```python
from build123d import *

# Parameters (mm, degrees)
SKETCH1_W           = 73.5
SKETCH1_H           = 5
BOSS_EXTRUDE1_DEPTH = 17
CUT_EXTRUDE1_DEPTH  = 195.359872402


with BuildPart() as part:
    # Sweep3: sweep along a path in Sketch2
    with BuildLine(Plane(origin=(0, 0, 0), x_dir=(0, 0, -1), z_dir=(1, 0, 0))) as sweep3_path:
        Line((-73.8, 0), (-73.8, 86.85))
        Line((-73.8, 86.85), (-63.15, 97.5))
        Line((-63.15, 97.5), (63.15, 97.5))
        Line((63.15, 97.5), (73.8, 86.85))
        Line((73.8, 86.85), (73.8, 0))
    # Sketch1 → Sweep3 (sweep)
    with BuildSketch(Plane(origin=(0, 0, 0), x_dir=(1, 0, 0), z_dir=(0, 1, 0))):
        with Locations((-13.25, -73.8)):
            Rectangle(SKETCH1_W, SKETCH1_H)
    sweep(path=sweep3_path.line, transition=Transition.RIGHT)

    # Sketch5 → Boss-Extrude1 (add)
    with BuildSketch(Plane.ZY.offset(50)):
        Polygon((-76.3, 0), (-71.3, 0), (-71.3, 85.814466094), (-62.114466094, 95), (62.114466094, 95), (71.3, 85.814466094), (71.3, 0), (76.3, 0), (76.3, 87.885533906), (64.185533906, 100), (-64.185533906, 100), (-76.3, 87.885533906), align=None)
    extrude(amount=BOSS_EXTRUDE1_DEPTH)

    # Sketch6 → Cut-Extrude1 (cut, through all)
    with BuildSketch(Plane(origin=(0, 0, -76.3), x_dir=(-1, 0, 0), z_dir=(0, 0, -1))):
        Polygon((52.03, 0), (67, 27), (67, 0), align=None)
    extrude(amount=-CUT_EXTRUDE1_DEPTH, mode=Mode.SUBTRACT)


solid = part.part
```
Geometry: final body of the model. Coordinates: model frame, mm. A direction names the side the tool comes from. Round coordinates to 2 decimals unless told otherwise and drop trailing zeros. Order: outer loops, then holes, each group sorted by start corner. A loop starts at its lowest first (then second) coordinate and runs counter-clockwise, first axis right, second up. Notation, with made-up numbers: M 35,-2.5 L 72,-2.5 A15 ccw 72,25.5 Z; hole C 10.25,-1 d8. An arc over 180 degrees is marked long. Use one line per item in the form item = value. Start each with the question number.
Q1. Access query for faces 1 (the face through (-21, 44, 71.3)), 2 (the face through (-21, 100, 1)). Directions: +Z, -Z, +X, -X, +Y, -Y. A direction counts if a zero-diameter tool reaches every point of the face in a straight line with its end or side. Return the directions, or none.
Q2. Material intervals for line 1 (Z direction, x = 4, y = 11); line 2 (Y direction, x = -10, z = 12); line 3 (Z direction, x = -34, y = 93), sorted ascending. Write a range as [from, to].
Q3. Cut plane C-C (y = 74). Return loops of the section in (x, z), and give its area (3 significant figures).
Q4. Cut plane D-D (z = 5). Return loops of the section in (x, y).
Q5. Cut plane B-B (x = -5). Return loops of the section in (y, z), and give its area (3 significant figures).
Q6. Cut plane A-A (y = 91.5). Return loops of the section in (x, z).
Q7. Mould query, pull axis Z, two halves, no side actions, for faces 3 (the face through (-21.117, 90.472, 66.643)), 4 (the face through (-21, 43, 76.3)), 5 (the face through (-59.41, 13.31, -73.83)). Classes: +Z half, -Z half, draft (parallel to the pull), parting line (faces both ways), or undercut.
Geometry results:
q1.face_1 = +X, -X, -Y
q1.face_2 = +Z, -Z, +X, -X, +Y
q2.line_1 = [-76.3, -71.3], [71.3, 76.3]
q2.line_2 = [95, 100]
q2.line_3 = [-71.19, -64.11], [64.11, 71.19]
q3.outline = M -67,-76.3 L 23.5,-76.3 L 23.5,-71.3 L -67,-71.3 Z; M -67,71.3 L 23.5,71.3 L 23.5,76.3 L -67,76.3 Z
q3.area = 905 mm^2
q4.outline = M -67,95 L 23.5,95 L 23.5,100 L -67,100 Z
q5.outline = M 0,-76.3 L 87.89,-76.3 L 100,-64.19 L 100,64.19 L 87.89,76.3 L 0,76.3 L 0,71.3 L 85.81,71.3 L 95,62.11 L 95,-62.11 L 85.81,-71.3 L 0,-71.3 Z
q5.area = 1,650 mm^2
q6.outline = M -67,-72.69 L 23.5,-72.69 L 23.5,-65.61 L -67,-65.61 Z; M -67,65.61 L 23.5,65.61 L 23.5,72.69 L -67,72.69 Z
q7.face_3 = undercut
q7.face_4 = +Z half
q7.face_5 = draft
